Here's how the part is built. I have some questions about the finished solid (model axes, mm). Face numbers are marked on the shaded views. Give positions to 0.01 mm unless a question says otherwise; leave off trailing zeros. Write each loop counter-clockwise with the first axis right and the second up, starting at its lowest first coordinate (ties: lowest second). Pieces come first, ordered by that corner, then holes. Notation, with made-up numbers: (70, -28) - (115, -28) arc R36 ccw to (115, 11) - close; hole circle Ø3 at (88, -10.75). An arc over 180 degrees is marked (long way). Use a Markdown table: item, result.
```python
from build123d import *

# Parameters (mm, degrees)
SKIZZE1_R                       = 10
SKIZZE1_R_2                     = 5.3
AUFSATZ_LINEAR_AUSTRAGEN1_DEPTH = 44
SKIZZE2_R                       = 5.5
SCHNITT_LINEAR_AUSTRAGEN1_DEPTH = 5.6
SKIZZE3_R                       = 5.894998856
SCHNITT_LINEAR_AUSTRAGEN2_DEPTH = 5.6
FASE1_SIZE                      = 0.4


with BuildPart() as part:
    # Skizze1 → Aufsatz-Linear austragen1 (new body)
    with BuildSketch(Plane.XY):
        Circle(SKIZZE1_R)
        Circle(SKIZZE1_R_2, mode=Mode.SUBTRACT)
    extrude(amount=AUFSATZ_LINEAR_AUSTRAGEN1_DEPTH)

    # Skizze2 → Schnitt-Linear austragen1 (cut)
    with BuildSketch(Plane.XY.offset(44)):
        Circle(SKIZZE2_R)
    extrude(amount=-SCHNITT_LINEAR_AUSTRAGEN1_DEPTH, mode=Mode.SUBTRACT)

    # Skizze3 → Schnitt-Linear austragen2 (cut)
    with BuildSketch(Plane(origin=(0, 0, 0), x_dir=(-1, 0, 0), z_dir=(0, 0, -1))):
        Circle(SKIZZE3_R)
    extrude(amount=-SCHNITT_LINEAR_AUSTRAGEN2_DEPTH, mode=Mode.SUBTRACT)

    # Fase1
    fase1_edges = [part.edges().sort_by_distance(p)[0] for p in [
        (-5.5, 0, 44),
        (5.894998856, 0, 0),
    ]]
    chamfer(fase1_edges, length=FASE1_SIZE)


solid = part.part
```
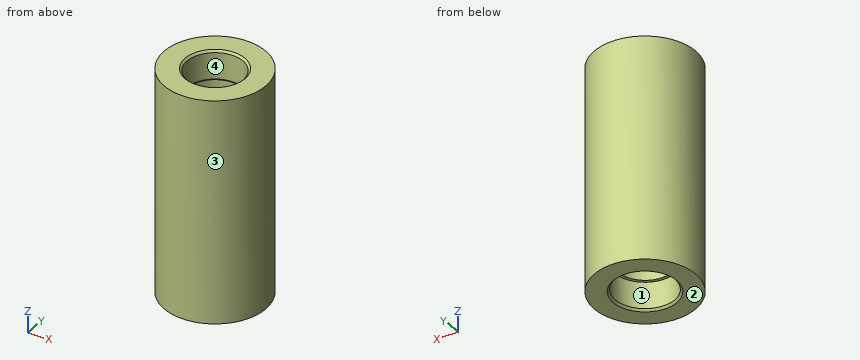
Item 1: If we section it at C-C, the plane z = 10: Write out the boundary of the cut face in (x, y).
Values:
| item | result |
|---|---|
| outline | circle Ø20 at (0, 0); hole circle Ø10.6 at (0, 0) |
Item 2: Thinking about a two-plate mould opening in X: for the marked faces 1, 2, 3 and 4, which applies, +X half, -X half, draft (parallel to the pull), parting line (faces both ways), or undercut?
Values:
| item | result |
|---|---|
| face 1 | undercut |
| face 2 | draft |
| face 3 | parting line |
| face 4 | undercut |
Item 3: I need wall thicknesses on line 1 along Y through (x, z) = (0, 26); line 2 along Y through (x, z) = (0, 41.6); line 3 along X through (y, z) = (-3, 26). Which ranges of each line are inside material? Lowest first, please. Write a range as [from, to].
Values:
| item | result |
|---|---|
| line 1 | y = [-10, -5.3], [5.3, 10] |
| line 2 | y = [-10, -5.5], [5.5, 10] |
| line 3 | x = [-9.54, -4.37], [4.37, 9.54] |
Item 4: If we section it at D-D, the plane x = 8: Write out the boundary of the cut face in (y, z).
Values:
| item | result |
|---|---|
| outline | (-6, 0) - (6, 0) - (6, 44) - (-6, 44) - close |
Item 5: If we section it at A-A, the plane x = 0: Write out the boundary of the cut face in (y, z) (3 decimals).
Values:
| item | result |
|---|---|
| outline | (-10, 0) - (-6.295, 0) - (-5.895, 0.4) - (-5.895, 5.6) - (-5.3, 5.6) - (-5.3, 38.4) - (-5.5, 38.4) - (-5.5, 43.6) - (-5.9, 44) - (-10, 44) - close; (5.3, 5.6) - (5.895, 5.6) - (5.895, 0.4) - (6.295, 0) - (10, 0) - (10, 44) - (5.9, 44) - (5.5, 43.6) - (5.5, 38.4) - (5.3, 38.4) - close |
Item 6: Will these pins go through, and if not, where does the flat tip stop? pin 1 Ø3 at (x, z) = (-6.5, 9.5) entering from +Y; pin 2 Ø6.5 at (x, y) = (0, 0) entering from -Z; pin 3 Ø4 at (x, z) = (7, 14.5) entering from -Y; pin 4 Ø9 at (x, y) = (-1, -0.5) entering from +Z.
Values:
| item | result |
|---|---|
| pin 1 | stops at y = 8.66 |
| pin 2 | passes through |
| pin 3 | stops at y = -8.66 |
| pin 4 | stops at z = 43.72 |
